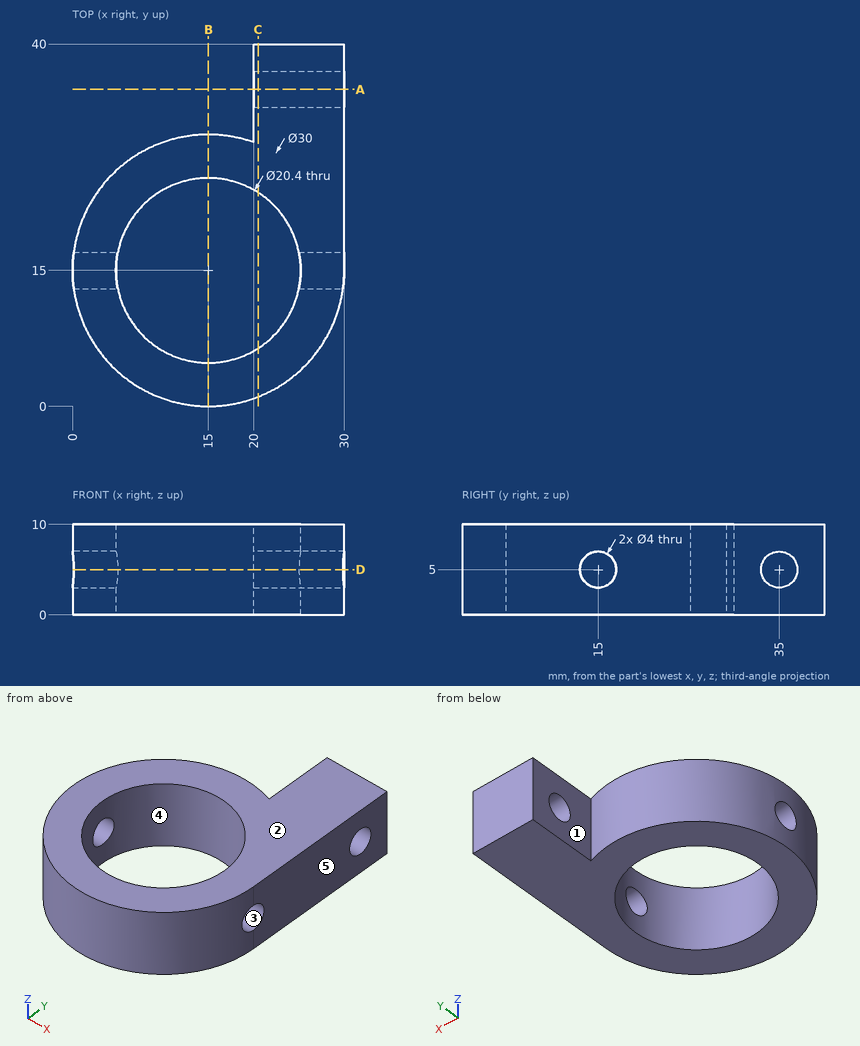
Source: three-view drawing plus pictorial views. Frame: mm from the lowest corner of the part. A direction names the side the tool comes from. Give positions to 0.01 mm unless a question says otherwise; leave off trailing zeros. Order: outer loops, then holes, each group sorted by start corner. A loop starts at its lowest first (then second) coordinate and runs counter-clockwise, first axis right, second up. Notation, with made-up numbers: M 84,31.5 L 96,31.5 A30 ccw 96,64.5 Z; hole C 20.5,58.25 d7. An arc over 180 degrees is marked long. Return JSON: item names as keys, results as strings.
Item 1: First-contact query: P1, Ø8, axis at x = 8, y = 33, coming from the +Z side; P2, Ø1, axis at y = 21.5, z = 3, coming from the -X side; P3, Ø4, axis at y = 9.5, z = 9, coming from the +X side; P4, Ø5, axis at y = 8, z = 7, coming from the +X side. Flat tips, straight axial feed; report the tip coordinate or a pass-through.
Solutions:
{"P1": "through", "P2": "x = 1.25", "P3": "x = 29.59", "P4": "x = 29.31"}
Item 2: Cut plane D-D (z = 5). Return loops of the section in (x, y), then the cut area to 3 significant figures.
Solutions:
{"outline": "M 0.13,13 A15 ccw 29.87,13 L 25,13 A10.2 cw 5,13 Z; M 0.13,17 L 5,17 A10.2 cw 25,17 L 30,17 L 30,33 L 20,33 L 20,29.14 A15 ccw Z; M 20,37 L 30,37 L 30,40 L 20,40 Z", "area": "448 mm^2"}
Item 3: Access query for the marked faces 1 and 2. Directions: +Z, -Z, +X, -X, +Y, -Y. A direction counts if a zero-diameter tool reaches every point of the face in a straight line with its end or side. Return the directions, or none.
Solutions:
{"face 1": "+Z, -Z, +Y", "face 2": "+Z, +X, -X, +Y, -Y"}
Item 4: Cut plane C-C (x = 20.5). Return loops of the section in (y, z).
Solutions:
{"outline": "M 1.04,0 L 6.41,0 L 6.41,10 L 1.04,10 Z; M 23.59,0 L 40,0 L 40,10 L 23.59,10 Z; hole C 35,5 d4"}
Item 5: Cut plane B-B (x = 15). Return loops of the section in (y, z).
Solutions:
{"outline": "M 0,0 L 4.8,0 L 4.8,10 L 0,10 Z; M 25.2,0 L 30,0 L 30,10 L 25.2,10 Z"}
Item 6: Pull-direction query (X, two-part tool) for the marked faces 3, 4 and 5; classes: +X half, -X half, draft (parallel to the pull), parting line (faces both ways), or undercut.
Solutions:
{"face 3": "draft", "face 4": "undercut", "face 5": "+X half"}
Item 7: Ray query, probe 1 along Y at (x, z) = (15, 4.25); probe 2 along Y at (x, z) = (27.3, 5); probe 3 along Y at (x, z) = (24, 5). Return the intervals inside material, ascending.
Solutions:
{"probe 1": "0 to 4.8, 25.2 to 30", "probe 2": "6.41 to 13, 17 to 33, 37 to 40", "probe 3": "3 to 10.2, 19.8 to 33, 37 to 40"}
Item 8: Cut plane A-A (y = 35). Return loops of the section in (x, z).
Solutions:
{"outline": "M 20,0 L 30,0 L 30,3 L 20,3 Z; M 20,7 L 30,7 L 30,10 L 20,10 Z"}
